Can you work these out from the drawing? Everything is in mm from the part's minimum corner. Coordinates: 2 decimals unless noted, no trailing zeros. Order: outer loops, then holes, each group sorted by start corner. A loop starts at its lowest first (then second) coordinate and runs counter-clockwise, first axis right, second up. Notation, with made-up numbers: (-18.5, 9.25) - (35.5, 9.25) arc R19 ccw to (35.5, 30.25) - close; hole circle Ø1 at (55, 37.5). An arc over 180 degrees is marked (long way). Use a Markdown table: item, result. Add a question column.
(1) If I drill on L1, parallel to Z at x = 27.5, y = 1.55; L2, parallel to X at y = 1.3, z = 30; L3, parallel to X at y = 2.4, z = 4, over which ranges is the centre line in solid material (lowest first)? Write a range as [from, to].
(2) I want a section at B-B (y = 1.65). List the corners of the cut face in (x, z) for me, and give its area (3 significant figures).
(3) I want a section at C-C (z = 33). List the corners of the cut face in (x, y) for me, and give its area (3 significant figures).
(4) For pin 1 Ø0.9 at (x, y) = (114, 1) entering from +Z; pin 2 Ø1.5 at (y, z) = (2, 28.5) entering from -X; pin 3 Ø0.9 at (x, y) = (1, 1) entering from +Z; pin 4 Ø1.5 at (y, z) = (1.5, 42) entering from +X, each with a flat end and sliding along its axis, tell me the tip position at first contact or that it passes through.
(5) I want a section at D-D (z = 7). List the corners of the cut face in (x, y) for me, and give its area (3 significant figures).
(6) I want a section at A-A (x = 67.5). List the corners of the cut face in (y, z) for me, and give its area (3 significant figures).
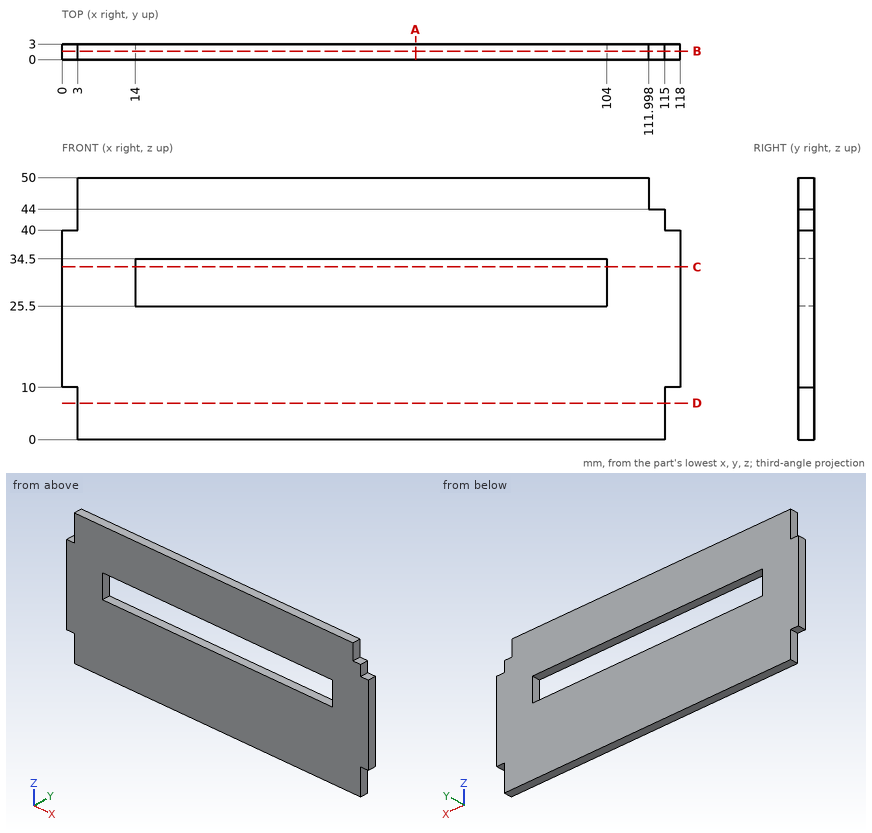
Answers follow:
| question | item | result |
|---|---|---|
| 1 | L1 | z = [0, 25.5], [34.5, 50] |
| 1 | L2 | x = [0, 14], [104, 118] |
| 1 | L3 | x = [3, 115] |
| 2 | outline | (0, 10) - (3, 10) - (3, 0) - (115, 0) - (115, 10) - (118, 10) - (118, 40) - (115, 40) - (115, 44) - (112, 44) - (112, 50) - (3, 50) - (3, 40) - (0, 40) - close; hole (14, 25.5) - (104, 25.5) - (104, 34.5) - (14, 34.5) - close |
| 2 | area | 4,950 mm² |
| 3 | outline | (0, 0) - (14, 0) - (14, 3) - (0, 3) - close; (104, 0) - (118, 0) - (118, 3) - (104, 3) - close |
| 3 | area | 84.0 mm² |
| 4 | pin 1 | stops at z = 44 |
| 4 | pin 2 | stops at x = 0 |
| 4 | pin 3 | stops at z = 40 |
| 4 | pin 4 | stops at x = 115 |
| 5 | outline | (3, 0) - (115, 0) - (115, 3) - (3, 3) - close |
| 5 | area | 336 mm² |
| 6 | outline | (0, 0) - (3, 0) - (3, 25.5) - (0, 25.5) - close; (0, 34.5) - (3, 34.5) - (3, 50) - (0, 50) - close |
| 6 | area | 123 mm² |
